Autodesk Inventor part; units mm, degrees
ref_plane "Work Plane1" through (47, 0, -94) normal (-1, 0, 0) x (0, 0, 1)
ref_plane "YZ Plane" through (0, 0, 0) normal (1, 0, 0) x (0, 1, 0)
ref_plane "XZ Plane" through (0, 0, 0) normal (0, 1, 0) x (-1, 0, 0)
sketch "Sketch3" plane through (0, 0, 0) normal (0, 1, 0) x (-1, 0, 0)
  line L0 (3, 3) -> (-97, 3) construction
  line L1 (-97, 3) -> (-97, 0) construction
  line L2 (-97, 0) -> (3, 0) construction
  line L3 (3, 0) -> (3, 3) construction
  line L4 (-97, 0) -> (-94, 0) construction
  line L5 (-94, 0) -> (-94, -94) construction
  line L6 (-94, -94) -> (-97, -94) construction
  line L7 (-97, -94) -> (-97, 0) construction
  line L8 (-97, -94) -> (3, -94) construction
  line L9 (3, -94) -> (3, -97) construction
  line L10 (3, -97) -> (-97, -97) construction
  line L11 (-97, -97) -> (-97, -94) construction
  line L12 (3, -94) -> (0, -94) construction
  line L13 (0, -94) -> (0, 0) construction
  line L14 (0, 0) -> (3, 0) construction
  line L15 (3, 0) -> (3, -94) construction
  line L16 (0, -94) -> (-94, -94)
  line L17 (-94, -94) -> (-94, 0)
  line L18 (-94, 0) -> (0, 0)
  line L19 (0, 0) -> (0, -94)
  line L20 (3, 3) -> (3, 0) construction
  dimension "d6" = 3
  dimension "d7" = 100
  dimension "d8" = 100
  dimension "d9" = 3
extrude "Extrusion2" add sketch "Sketch3" along normal blind 3
sketch "Sketch4" plane through (0, 3, 0) normal (0, 1, 0) x (1, 0, 0)
  line L0 (94, 94) -> (0, 94)
  line L1 (0, 0) -> (94, 0)
  line L2 (0, 94) -> (5, 94)
  line L3 (5, 94) -> (5, 0)
  line L4 (5, 0) -> (0, 0)
  line L5 (0, 0) -> (0, 94)
  line L6 (94, 0) -> (94, 94)
  line L7 (94, 94) -> (89, 94)
  line L8 (89, 94) -> (89, 0)
  line L9 (89, 0) -> (94, 0)
  line L10 (94, 0) -> (94, 94)
  line L11 (5, 3) -> (89, 3)
  line L12 (89, 3) -> (89, 0)
  line L13 (89, 0) -> (5, 0)
  line L14 (5, 0) -> (5, 3)
  dimension "d12" = 5
  dimension "d13" = 3
extrude "Extrusion3" add sketch "Sketch4" along normal blind 5 contours L6 L1 L8 L0 | L3 L1 L5 L0 | L8 L1 L3 L11
sketch "Sketch6" plane through (94, 0, -94) normal (0, 0, -1) x (-1, 0, 0)
  line L0 (0, 0) -> (94, 0)
  line L1 (89, 8) -> (94, 8)
  line L2 (89, 3) -> (89, 8)
  line L3 (94, 0) -> (94, 8)
  line L4 (0, 0) -> (0, 8)
  point P0 (91.5, 4)
  point P1 (2.5, 4)
  dimension "d28" = 8
  dimension "d29" = 5
  dimension "d30" = 2.5
  dimension "d31" = 4
  dimension "d32" = 2.5
hole "Hole1" at (2.5, 4, -94) at (91.5, 4, -94) direction (0, 0, 1) diameter 2.6416 depth 10.979 tip angle 118
fillet "Fillet1" radius 3 2 edges at (89, 5.5, -3) (5, 5.5, -3)
fillet "Fillet2" radius 0.5 2 edges at (5, 5.5, -94) (89, 5.5, -94)
sketch "Sketch7" plane through (0, 0, 0) normal (0, 0, 1) x (1, 0, 0)
  line L0 (0, 0) -> (94, 0)
  line L1 (0, 0) -> (0, 8)
  line L2 (89, 8) -> (5, 8)
  point P0 (19, 4)
  point P1 (47, 4)
  point P2 (75, 4)
  dimension "d40" = 4
  dimension "d57" = 84
  dimension "d58" = 14
  dimension "d59" = 28
  dimension "d60" = 28
hole "Hole2" at (19, 4, 0) at (47, 4, 0) at (75, 4, 0) direction (0, 0, -1) diameter 2.459 depth 3.5 tip angle 118
sketch "Sketch9" plane through (0, 0, -94) normal (-1, 0, 0) x (0, 0, 1)
  line L0 (0, 8) -> (94, 8)
  line L1 (0, 0) -> (94, 0)
  line L2 (0, 0) -> (0, 8)
  point P0 (23.5, 4)
  point P1 (70.5, 4)
  dimension "d51" = 4
  dimension "d52" = 8
  dimension "d53" = 94
  dimension "d54" = 23.5
  dimension "d55" = 47
hole "Hole3" at (0, 4, -70.5) at (0, 4, -23.5) direction (1, 0, 0) diameter 2.459 depth 4 tip angle 118
ref_plane "Work Plane1" through (47, 0, -94) normal (-1, 0, 0) x (0, 0, 1)
mirror "Mirror1" about plane through (47, 0, -94) normal (-1, 0, 0) of "Hole3"
chamfer "Chamfer2" distance 1 angle 45 1 edges at (47, 3, -94)
chamfer "Chamfer3" distance 0.5 angle 45 3 edges at (5, 8, -49.75) (47, 8, -3) (89, 8, -49.75)
ref_plane "Work Plane2" through (47, 0, -94) normal (-1, 0, 0) x (0, 0, 1)
properties part number "LeftPanel" material "Aluminum 6061"
Model file for the job. Use its own axes, mm. A direction names the side the tool comes from. Round coordinates to 2 decimals unless told otherwise and drop trailing zeros. Order: outer loops, then holes, each group sorted by start corner. A loop starts at its lowest first (then second) coordinate and runs counter-clockwise, first axis right, second up. Notation, with made-up numbers: M 13.5,-13 L 24.5,-13 A11 ccw 24.5,-4 Z; hole C 36,44.25 d3. An arc over 180 degrees is marked long. Write each question's results on one line, items separated by ' | '. Start each with the question number.
(1) Two-plate mould, pull along Z, no slides. Class faces 4 (the face through (46.8, 1.8, -94)), 5 (the face through (2.028, 4.471, -22.364)), 6 (the face through (46.631, 2.827, -1.774)), 7 (the face through (89.39, 3.991, -70.713)): pulls with the +Z half, pulls with the -Z half, needs draft (parallel to the pull), parting line crosses it, or undercut.
(2) Saw through at B-B, the plane z = -41. Give the cut face in (x, y).
(3) Drop flat-ended pins along their axis: pin 1 (4 mm diameter, centred on x = 67, z = -83.5, fed in from +Y); pin 2 (3 mm diameter, centred on x = 47, y = 4, fed in from -Z); pin 3 (2 mm diameter, centred on y = 4, z = -70.5, fed in from -X). Give the stop position or say it passes through.
(4) Saw through at A-A, the plane x = 25. Give the cut face in (y, z), then the cut area to 3 significant figures.
(5) Probe probe 1 along X at (y, z) = (4, -85.75); probe 2 along Z at (x, y) = (1.05, 4). List the from-to ranges inside material, lowest first. Write a range as from..to.
(6) Which spindle directions (+Z, -Z, +X, -X, +Y, -Y) get a long thin tool onto all of the face, cutting with end or side? Do faces 1 (the face through (3.01, 5.22, -88.43)), 2 (the face through (0, 4, -46)), 3 (the face through (88.1, 5.28, -3.86)). Say none if no direction does.
Established:
1) face 4: pulls with the -Z half | face 5: undercut | face 6: needs draft | face 7: undercut
2) outline: M 0,0 L 94,0 L 94,8 L 89.5,8 L 89,7.5 L 89,3 L 5,3 L 5,7.5 L 4.5,8 L 0,8 Z
3) pin 1: stops at y = 3 | pin 2: stops at z = -93.5 | pin 3: stops at x = 4.14
4) outline: M 0,-94 L 2,-94 L 3,-93 L 3,-3 L 7.5,-3 L 8,-2.5 L 8,0 L 0,0 Z | area: 296 mm^2
5) probe 1: x = 0..1.18, 3.82..5, 89..90.18, 92.82..94 | probe 2: z = -94..-71.73, -69.27..-24.73, -22.27..0
6) face 1: -Z | face 2: +Z, -Z, -X, +Y, -Y | face 3: -Z, +Y
